CAD build for the part. Positions are in the model's coordinates, mm. A direction names the side the tool comes from. Coordinates: 2 decimals unless noted, no trailing zeros. Loops run counter-clockwise (first coordinate to the right, second up) from the corner with the lowest first, then second, coordinate; pieces in that order, holes last. Notation, with made-up numbers: (22.25, -26) - (62.25, -26) arc R23 ccw to (62.25, -11) - close; hole circle Ø2 at (14.5, -33). An arc over 180 degrees is marked (long way). Put each result on its own line as item: value.
```python
from build123d import *

# Parameters (mm, degrees)
SKETCH_W      = 1.9
SKETCH_H      = 5
PAD_DEPTH     = 90
SKETCH001_W   = 2
SKETCH001_H   = 69
SKETCH001_H_2 = 73
POCKET_DEPTH  = 5
SKETCH002_W   = 60.2
SKETCH002_H   = 11.5
PAD001_DEPTH  = 2
SKETCH004_W   = 2
SKETCH004_H   = 2
PAD002_DEPTH  = 4


with BuildPart() as part:
    # Sketch → Pad (new body)
    with BuildSketch(Plane.XZ):
        Polygon((-30.1, 0), (30.1, 0), (30.1, 15.5), (28.1, 15.5), (28.1, 2), (-28.1, 2), (-28.1, 15.5), (-30.1, 15.5), align=None)
        with Locations((0, 4.5)):
            Rectangle(SKETCH_W, SKETCH_H)
        with Locations((-20.05, 4.5)):
            Rectangle(SKETCH_W, SKETCH_H)
        with Locations((20.05, 4.5)):
            Rectangle(SKETCH_W, SKETCH_H)
    extrude(amount=PAD_DEPTH)

    # Sketch001 (on Face3 of Pad) → Pocket (cut)
    with BuildSketch(Plane(origin=(0, 0, 15.5), x_dir=(-1, 0, 0), z_dir=(0, 0, 1))):
        with Locations((29.1, 55.5)):
            Rectangle(SKETCH001_W, SKETCH001_H)
        with Locations((-29.1, 53.5)):
            Rectangle(SKETCH001_W, SKETCH001_H_2)
    extrude(amount=-POCKET_DEPTH, mode=Mode.SUBTRACT)

    # Sketch002 (on Face2 of Pocket) → Pad001 (join)
    with BuildSketch(Plane(origin=(0, 0, 0), x_dir=(1, 0, 0), z_dir=(0, 1, 0))):
        with Locations((0, -5.75)):
            Rectangle(SKETCH002_W, SKETCH002_H)
    extrude(amount=PAD001_DEPTH)

    # Sketch004 → Pad002 (join)
    with BuildSketch(Plane(origin=(0, 0, 11.5), x_dir=(-1, 0, 0), z_dir=(0, 0, 1))):
        with Locations((-29.1, -1)):
            Rectangle(SKETCH004_W, SKETCH004_H)
        with Locations((29.1, -1)):
            Rectangle(SKETCH004_W, SKETCH004_H)
    extrude(amount=PAD002_DEPTH)


solid = part.part
```
Q1. Slice it at A-A, the plane z = 12.75. Give the cut face in (x, y).
Determined:
outline: (-30.1, -21) - (-28.1, -21) - (-28.1, 2) - (-30.1, 2) - close; (28.1, -17) - (30.1, -17) - (30.1, 2) - (28.1, 2) - close
Q2. Tool access for faces 1 (the flat face through (-20, -44, 7)), 2 (the flat face through (0, -90, 3)), 3 (the flat face through (-29, -21, 13)): list every direction of +Z, -Z, +X, -X, +Y, -Y with a clear straight run to the whole face (end or side of a thin tool).
Determined:
face 1: +Z, -Y
face 2: +Z, -Z, +X, -X, -Y
face 3: +Z, +X, -X, -Y
Q3. Slice it at B-B, the plane y = -4. Give the cut face in (x, z), then the cut area to 3 significant figures.
Determined:
outline: (-30.1, 0) - (30.1, 0) - (30.1, 15.5) - (28.1, 15.5) - (28.1, 2) - (21, 2) - (21, 7) - (19.1, 7) - (19.1, 2) - (0.95, 2) - (0.95, 7) - (-0.95, 7) - (-0.95, 2) - (-19.1, 2) - (-19.1, 7) - (-21, 7) - (-21, 2) - (-28.1, 2) - (-28.1, 15.5) - (-30.1, 15.5) - close
area: 203 mm2
Q4. Slice it at D-D, the plane x = 8. Give the cut face in (y, z).
Determined:
outline: (-90, 0) - (2, 0) - (2, 11.5) - (0, 11.5) - (0, 2) - (-90, 2) - close
Q5. Pin check, flat tips, straight feed: pin 1 Ø1 at (x, z) = (29, 13.5) entering from -Y; pin 2 Ø9 at (x, y) = (7, -39.5) entering from +Z; pin 3 Ø7 at (y, z) = (-57.5, 11.5) entering from -X; pin 4 Ø5 at (x, z) = (-4, 5) entering from -Y. Stop position of each tip, or through.
Determined:
pin 1: y = -17
pin 2: z = 2
pin 3: x = -30.1
pin 4: y = 0
Q6. Wall check: L1, parallel to X at y = -26.5, z = 3; L2, parallel to X at y = -83, z = 9.5; L3, parallel to Y at x = -20.5, z = 10.5. Give the ranges that are in metal, low to high. Write a range as from..to.
Determined:
L1: -30.1..-28.1, -21..-19.1, -0.95..0.95, 19.1..21, 28.1..30.1
L2: -30.1..-28.1, 28.1..30.1
L3: 0..2
Q7. Slice it at C-C, the plane z = 4.5. Give the cut face in (x, y).
Determined:
outline: (-30.1, -90) - (-28.1, -90) - (-28.1, 0) - (-21, 0) - (-21, -90) - (-19.1, -90) - (-19.1, 0) - (-0.95, 0) - (-0.95, -90) - (0.95, -90) - (0.95, 0) - (19.1, 0) - (19.1, -90) - (21, -90) - (21, 0) - (28.1, 0) - (28.1, -90) - (30.1, -90) - (30.1, 2) - (-30.1, 2) - close
